Input: part model. Units: mm. Frame: model coordinates. A direction names the side the tool comes from. Coordinates: 2 decimals unless noted, no trailing zeros. Order: outer loops, then holes, each group sorted by start corner. A loop starts at its lowest first (then second) coordinate and runs counter-clockwise, first axis right, second up. Notation, with made-up numbers: (-11, -3.5) -> (0, -3.5) arc R23 cw to (0, 27.5) -> close; hole circle Ø4 at (38.5, 36). An arc over 180 degrees is marked (long way). One line per question, with ' | ' between items.
```python
from build123d import *

# Parameters (mm, degrees)
F0_W           = 60
F0_H           = 40
F1_DEPTH       = 2.2
F2_D           = 4.25
F2_DEPTH       = 15
F2_CSINK_D     = 7
F2_CSINK_ANGLE = 90
F2_TIP         = 1.2768288154
F3_R           = 3
F4_W           = 50
F4_H           = 20
F5_DEPTH       = 1
F6_R           = 5
F7_T4_ANGLE    = 90
F7_T9_DEPTH    = 40
F7_T14_DEPTH   = 22.7150489639
F7_T19_ANGLE   = 90
F7_T24_DEPTH   = 22.7150489639
F9_DEPTH       = 0.4
F10_T4_ANGLE   = 90
F10_T9_DEPTH   = 40
F10_T14_DEPTH  = 15
F10_T19_ANGLE  = 90
F10_T24_DEPTH  = 15


# Not quite as in the source:
# - a fillet or chamfer that OpenCascade refuses, or shapes differently, is made with other operations: its cross-section is extruded or revolved along the edge and cut away or added


with BuildPart() as f1:
    # F0 (on Top) → F1 (new body)
    with BuildSketch(Plane.XY):
        Rectangle(F0_W, F0_H)
    extrude(amount=F1_DEPTH)

    # F2
    with Locations(Plane(origin=(0, 0, 0), x_dir=(1, 0, 0), z_dir=(0, 0, -1))):
        with Locations((-25, 15), (25, 15)):
            CounterSinkHole(F2_D / 2, F2_CSINK_D / 2, depth=F2_DEPTH, counter_sink_angle=F2_CSINK_ANGLE)
            with Locations((0, 0, -(F2_DEPTH + F2_TIP / 2))):  # 118° drill point
                Cone(0, F2_D / 2, F2_TIP, mode=Mode.SUBTRACT)

    # F3
    f3_edges = [f1.edges().sort_by_distance(p)[0] for p in [
        (-30, -20, 1.1),
        (30, -20, 1.1),
    ]]
    fillet(f3_edges, radius=F3_R)

    # F4 (on face) → F5 (cut)
    with BuildSketch(Plane.XY.offset(2.2)):
        with Locations((0, 10)):
            Rectangle(F4_W, F4_H)
    extrude(amount=-F5_DEPTH, mode=Mode.SUBTRACT)

    # F6
    f6_edges = [f1.edges().sort_by_distance(p)[0] for p in [
        (25, 0, 1.7),
        (-25, 0, 1.7),
    ]]
    fillet(f6_edges, radius=F6_R)

    # F7: chamfer of 3 on 1 edges, made by hand


with BuildPart() as f7_tool2:
    # F7_s3 → F7_t4 (revolve)
    with BuildSketch(Plane.YZ.offset(20)):
        Polygon((-3, 2.2), (0, -0.8), (0, 2.2), align=None)
    revolve(axis=Axis((20, 5, 2.2), (0, 0, 1)), revolution_arc=F7_T4_ANGLE)

    split(bisect_by=Plane.XY.offset(1.2), keep=Keep.TOP)


with BuildPart() as f1_1:
    add(f1.part)

    # F7_t1: cut F7_tool2
    add(f7_tool2.part, mode=Mode.SUBTRACT)


with BuildPart() as f7_tool7:
    # F7_s8 → F7_t9 (new body)
    with BuildSketch(Plane.YZ.offset(-20)):
        Polygon((-3, 2.2), (0, -0.8), (0, 2.2), align=None)
    extrude(amount=F7_T9_DEPTH)

    split(bisect_by=Plane.XY.offset(1.2), keep=Keep.TOP)


with BuildPart() as f1_2:
    add(f1_1.part)

    # F7_t6: cut F7_tool7
    add(f7_tool7.part, mode=Mode.SUBTRACT)


with BuildPart() as f7_tool12:
    # F7_s13 → F7_t14 (new body)
    with BuildSketch(Plane.XZ.offset(-5)):
        Polygon((28, 2.2), (25, -0.8), (25, 2.2), align=None)
    extrude(amount=-F7_T14_DEPTH)

    split(bisect_by=Plane.XY.offset(1.2), keep=Keep.TOP)


with BuildPart() as f1_3:
    add(f1_2.part)

    # F7_t11: cut F7_tool12
    add(f7_tool12.part, mode=Mode.SUBTRACT)


with BuildPart() as f7_tool17:
    # F7_s18 → F7_t19 (revolve)
    with BuildSketch(Plane.XZ.offset(-5)):
        Polygon((-28, 2.2), (-25, -0.8), (-25, 2.2), align=None)
    revolve(axis=Axis((-20, 5, 2.2), (0, 0, 1)), revolution_arc=F7_T19_ANGLE)

    split(bisect_by=Plane.XY.offset(1.2), keep=Keep.TOP)


with BuildPart() as f1_4:
    add(f1_3.part)

    # F7_t16: cut F7_tool17
    add(f7_tool17.part, mode=Mode.SUBTRACT)


with BuildPart() as f7_tool22:
    # F7_s23 → F7_t24 (new body)
    with BuildSketch(Plane.XZ.offset(-27.7150489639)):
        Polygon((-28, 2.2), (-25, -0.8), (-25, 2.2), align=None)
    extrude(amount=F7_T24_DEPTH)

    split(bisect_by=Plane.XY.offset(1.2), keep=Keep.TOP)


with BuildPart() as f1_5:
    add(f1_4.part)

    # F7_t21: cut F7_tool22
    add(f7_tool22.part, mode=Mode.SUBTRACT)

    # F8 (on face) → F9 (cut)
    with BuildSketch(Plane.XY.offset(1.2)):
        with BuildLine():
            ThreePointArc((20, 3), (21.4142135624, 3.5857864376), (22, 5))
            Line((22, 5), (22, 20))
            Line((22, 20), (-22, 20))
            Line((-22, 20), (-22, 5))
            ThreePointArc((-22, 5), (-21.4142135624, 3.5857864376), (-20, 3))
            Line((-20, 3), (20, 3))
        make_face()
    extrude(amount=-F9_DEPTH, mode=Mode.SUBTRACT)

    # F10: chamfer of 1 on 1 edges, made by hand


with BuildPart() as f10_tool2:
    # F10_s3 → F10_t4 (revolve)
    with BuildSketch(Plane.YZ.offset(20)):
        Polygon((4, 0.8), (3, 1.8), (3, 0.8), align=None)
    revolve(axis=Axis((20, 5, 0.8), (0, 0, 1)), revolution_arc=F10_T4_ANGLE)

    split(bisect_by=Plane.XY.offset(1.2), keep=Keep.BOTTOM)


with BuildPart() as f1_6:
    add(f1_5.part)

    # F10_t1: union F10_tool2
    add(f10_tool2.part)


with BuildPart() as f10_tool7:
    # F10_s8 → F10_t9 (new body)
    with BuildSketch(Plane.YZ.offset(-20)):
        Polygon((4, 0.8), (3, 1.8), (3, 0.8), align=None)
    extrude(amount=F10_T9_DEPTH)

    split(bisect_by=Plane.XY.offset(1.2), keep=Keep.BOTTOM)


with BuildPart() as f1_7:
    add(f1_6.part)

    # F10_t6: union F10_tool7
    add(f10_tool7.part)


with BuildPart() as f10_tool12:
    # F10_s13 → F10_t14 (new body)
    with BuildSketch(Plane.XZ.offset(-5)):
        Polygon((21, 0.8), (22, 1.8), (22, 0.8), align=None)
    extrude(amount=-F10_T14_DEPTH)

    split(bisect_by=Plane.XY.offset(1.2), keep=Keep.BOTTOM)


with BuildPart() as f1_8:
    add(f1_7.part)

    # F10_t11: union F10_tool12
    add(f10_tool12.part)


with BuildPart() as f10_tool17:
    # F10_s18 → F10_t19 (revolve)
    with BuildSketch(Plane.XZ.offset(-5)):
        Polygon((-21, 0.8), (-22, 1.8), (-22, 0.8), align=None)
    revolve(axis=Axis((-20, 5, 0.8), (0, 0, 1)), revolution_arc=F10_T19_ANGLE)

    split(bisect_by=Plane.XY.offset(1.2), keep=Keep.BOTTOM)


with BuildPart() as f1_9:
    add(f1_8.part)

    # F10_t16: union F10_tool17
    add(f10_tool17.part)


with BuildPart() as f10_tool22:
    # F10_s23 → F10_t24 (new body)
    with BuildSketch(Plane.XZ.offset(-20)):
        Polygon((-22, 1.8), (-21, 0.8), (-22, 0.8), align=None)
    extrude(amount=F10_T24_DEPTH)

    split(bisect_by=Plane.XY.offset(1.2), keep=Keep.BOTTOM)


with BuildPart() as f1_10:
    add(f1_9.part)

    # F10_t21: union F10_tool22
    add(f10_tool22.part)


solid = f1_10.part
```
1. Ray query, line 1 (X direction, y = -15, z = 1.6) (3 decimals); line 2 (Z direction, x = 23.5, y = 11.5); line 3 (Z direction, x = -19, y = 18). Return the intervals inside material, ascending. Write a range as [from, to].
Recorded:
line 1: x = [-30, -27.125], [-22.875, 22.875], [27.125, 30] | line 2: z = [0, 1.2] | line 3: z = [0, 0.8]
2. Pin query (flat end, axial travel): pin 1 Ø11 at (x, y) = (4, 10) entering from +Z; pin 2 Ø4 at (x, y) = (-25, -15) entering from -Z. Return the tip coordinate at first contact, or that it passes through.
Recorded:
pin 1: stops at z = 0.8 | pin 2: passes through
3. Cut plane B-B, the plane z = 1.8. Return loops of the section in (x, y) (3 decimals).
Recorded:
outline: (-30, -17) arc R3 ccw to (-27, -20) -> (27, -20) arc R3 ccw to (30, -17) -> (30, 20) -> (27.6, 20) -> (27.6, 5) arc R7.6 cw to (20, -2.6) -> (-20, -2.6) arc R7.6 cw to (-27.6, 5) -> (-27.6, 20) -> (-30, 20) -> close; hole circle Ø4.25 at (-25, -15); hole circle Ø4.25 at (25, -15)
4. Access query for faces 4 (the face through (20.81, 4.17, 0.96)), 5 (the face through (27.123, -15.093, 1.793)). Directions: +Z, -Z, +X, -X, +Y, -Y. A direction counts if a zero-diameter tool reaches every point of the face in a straight line with its end or side. Return the directions, or none.
Recorded:
face 4: +Z, +Y | face 5: +Z, -Z
5. Cut plane C-C, the plane y = 10.5. Return loops of the section in (x, z), and give its area (3 significant figures).
Recorded:
outline: (-30, 0) -> (30, 0) -> (30, 2.2) -> (28, 2.2) -> (27, 1.2) -> (21.4, 1.2) -> (21, 0.8) -> (-21, 0.8) -> (-21.4, 1.2) -> (-27, 1.2) -> (-28, 2.2) -> (-30, 2.2) -> close | area: 60.0 mm^2
6. Cut plane D-D, the plane x = 7. Return loops of the section in (y, z), and give its area (3 significant figures).
Recorded:
outline: (-20, 0) -> (20, 0) -> (20, 0.8) -> (4, 0.8) -> (3.6, 1.2) -> (-2, 1.2) -> (-3, 2.2) -> (-20, 2.2) -> close | area: 59.0 mm^2
7. Cut plane A-A, the plane y = -15. Return loops of the section in (x, z) (3 decimals), and give its area (3 significant figures).
Recorded:
outline: (-30, 0) -> (-28.5, 0) -> (-27.125, 1.375) -> (-27.125, 2.2) -> (-30, 2.2) -> close; (-22.875, 1.375) -> (-21.5, 0) -> (21.5, 0) -> (22.875, 1.375) -> (22.875, 2.2) -> (-22.875, 2.2) -> close; (27.125, 1.375) -> (28.5, 0) -> (30, 0) -> (30, 2.2) -> (27.125, 2.2) -> close | area: 110 mm^2
8. Mould query, pull axis Y, two halves, no side actions, for faces 1 (the face through (-22.877, -15.093, 1.793)), 2 (the face through (-25.118, -0.007, 1.36)), 3 (the face through (0, 12, 0.8)). Classes: released by +Y, released by -Y, zero draft, split by the parting line, or undercut.
Recorded:
face 1: undercut | face 2: released by +Y | face 3: zero draft
